Read the model definition and answer for the solid it produces. Units are mm, in the model's axes. A direction names the side the tool comes from. Coordinates: 2 decimals unless noted, no trailing zeros. Loops run counter-clockwise (first coordinate to the right, second up) from the corner with the lowest first, then second, coordinate; pieces in that order, holes last. Notation, with made-up numbers: (-32.5, 21.5) -> (-0.5, 21.5) arc R11 ccw to (-0.5, 30.5) -> close; hole circle Ø10 at (-27, 83). An arc over 180 degrees is marked (long way). Answer as a JSON object with one key per item and string values. Group by question number.
1) Which of the six approach directions +Z, -Z, +X, -X, +Y, -Y give full straight-line access (tool end or side, diameter ignored) to faces 1 (the face through (-72.52, -15, -21)), 2 (the face through (-76, -30, -42))?
2) Determine the mould class of faces 3 (the face through (-25.396, -15, -12)), 4 (the face through (-72.77, -14.79, -11.72)), 5 (the face through (-14.987, -15, -43)), 6 (the face through (-134.987, -15, -43)) for opening direction X: released by +X, released by -X, zero draft, split by the parting line, or undercut.
3) Section A-A, the plane x = -47 is taken. Give the vertices of the cut face in (y, z), plus the area to 3 significant figures.
4) Consider probe 1 along Z at (x, y) = (-119, -21.5); probe 2 along Z at (x, y) = (-49, -6); probe 3 along Z at (x, y) = (-87.5, -7.5). Determine where each line is inside the solid, lowest interval first. Write a range as [from, to].
5) Section B-B, the plane y = -4.5 is taken. Count the separate pieces of the cut face and the enclosed holes in it, plus the area to 3 significant figures.
from build123d import *

# Parameters (mm, degrees)
F0_W     = 120
F0_H     = 85
F0_W_2   = 6.2300768045
F0_H_2   = 1.9291306924
F1_DEPTH = 30


with BuildPart() as f1:
    # F0 (on Front) → F1 (new body)
    with BuildSketch(Plane.XZ):
        with Locations((-74.9865994975, -42.5)):
            Rectangle(F0_W, F0_H)
        with BuildLine():
            Line((-121.3085489491, -24.3586543947), (-121.3085489491, -5.8024477979))
            Line((-121.3085489491, -5.8024477979), (-116.0653747936, -5.8024477979))
            add(Edge.make_bspline(
                [(-116.0653747936, -5.8024477979), (-112.3736278476, -5.8024477979), (-110.7226981077, -6.9071289523)],
                knots=[0, 0, 0, 1, 1, 1], degree=2))
            add(Edge.make_bspline(
                [(-110.7226981077, -6.9071289523), (-109.0717683678, -8.0118101066), (-109.0717683678, -10.3958095096)],
                knots=[0, 0, 0, 1, 1, 1], degree=2))
            add(Edge.make_bspline(
                [(-109.0717683678, -10.3958095096), (-109.0717683678, -12.0487699134), (-109.9916591084, -13.1209604456)],
                knots=[0, 0, 0, 1, 1, 1], degree=2))
            add(Edge.make_bspline(
                [(-109.9916591084, -13.1209604456), (-110.9115498491, -14.1931509778), (-112.6782274306, -14.5099345441)],
                knots=[0, 0, 0, 1, 1, 1], degree=2))
            Line((-112.6782274306, -14.5099345441), (-112.6782274306, -14.6358357051))
            add(Edge.make_bspline(
                [(-112.6782274306, -14.6358357051), (-108.4503852184, -15.3587520488), (-108.4503852184, -19.0789282893)],
                knots=[0, 0, 0, 1, 1, 1], degree=2))
            add(Edge.make_bspline(
                [(-108.4503852184, -19.0789282893), (-108.4503852184, -21.5644608866), (-110.1317749166, -22.9615576407)],
                knots=[0, 0, 0, 1, 1, 1], degree=2))
            add(Edge.make_bspline(
                [(-110.1317749166, -22.9615576407), (-111.8131646148, -24.3586543947), (-114.8347924783, -24.3586543947)],
                knots=[0, 0, 0, 1, 1, 1], degree=2))
            Line((-114.8347924783, -24.3586543947), (-121.3085489491, -24.3586543947))
        make_face(mode=Mode.SUBTRACT)
        with BuildLine():
            add(Edge.make_bspline(
                [(-94.4976936528, -12.1360884606), (-92.7777213407, -14.0794338002), (-92.7777213407, -17.3894159355)],
                knots=[0, 0, 0, 1, 1, 1], degree=2))
            add(Edge.make_bspline(
                [(-92.7777213407, -17.3894159355), (-92.7777213407, -20.7928086097), (-94.4895709972, -22.7036633271)],
                knots=[0, 0, 0, 1, 1, 1], degree=2))
            add(Edge.make_bspline(
                [(-94.4895709972, -22.7036633271), (-96.2014206537, -24.6145180445), (-99.2230485172, -24.6145180445)],
                knots=[0, 0, 0, 1, 1, 1], degree=2))
            add(Edge.make_bspline(
                [(-99.2230485172, -24.6145180445), (-101.0912592929, -24.6145180445), (-102.5370919803, -23.7372712454)],
                knots=[0, 0, 0, 1, 1, 1], degree=2))
            add(Edge.make_bspline(
                [(-102.5370919803, -23.7372712454), (-103.9829246676, -22.8600244463), (-104.7708222557, -21.2233093536)],
                knots=[0, 0, 0, 1, 1, 1], degree=2))
            add(Edge.make_bspline(
                [(-104.7708222557, -21.2233093536), (-105.5587198437, -19.5865942609), (-105.5587198437, -17.3894159355)],
                knots=[0, 0, 0, 1, 1, 1], degree=2))
            add(Edge.make_bspline(
                [(-105.5587198437, -17.3894159355), (-105.5587198437, -13.9900845891), (-103.8570235067, -12.0914138551)],
                knots=[0, 0, 0, 1, 1, 1], degree=2))
            add(Edge.make_bspline(
                [(-103.8570235067, -12.0914138551), (-102.1553271696, -10.192743121), (-99.1336993061, -10.192743121)],
                knots=[0, 0, 0, 1, 1, 1], degree=2))
            add(Edge.make_bspline(
                [(-99.1336993061, -10.192743121), (-96.2176659648, -10.192743121), (-94.4976936528, -12.1360884606)],
                knots=[0, 0, 0, 1, 1, 1], degree=2))
        make_face(mode=Mode.SUBTRACT)
        with BuildLine():
            Line((-78.9651455832, -24.3586543947), (-80.528756776, -24.3586543947))
            Line((-80.528756776, -24.3586543947), (-80.9470735367, -22.3767264413))
            Line((-80.9470735367, -22.3767264413), (-81.048606731, -22.3767264413))
            add(Edge.make_bspline(
                [(-81.048606731, -22.3767264413), (-82.088306641, -23.6844739844), (-83.1219145593, -24.1494960144)],
                knots=[0, 0, 0, 1, 1, 1], degree=2))
            add(Edge.make_bspline(
                [(-83.1219145593, -24.1494960144), (-84.1555224777, -24.6145180445), (-85.7069496871, -24.6145180445)],
                knots=[0, 0, 0, 1, 1, 1], degree=2))
            add(Edge.make_bspline(
                [(-85.7069496871, -24.6145180445), (-87.7741655238, -24.6145180445), (-88.9478892503, -23.5463888401)],
                knots=[0, 0, 0, 1, 1, 1], degree=2))
            add(Edge.make_bspline(
                [(-88.9478892503, -23.5463888401), (-90.1216129769, -22.4782596356), (-90.1216129769, -20.5125769933)],
                knots=[0, 0, 0, 1, 1, 1], degree=2))
            add(Edge.make_bspline(
                [(-90.1216129769, -20.5125769933), (-90.1216129769, -16.3009800922), (-83.3838702007, -16.0979137036)],
                knots=[0, 0, 0, 1, 1, 1], degree=2))
            Line((-83.3838702007, -16.0979137036), (-81.0242387644, -16.0207484759))
            Line((-81.0242387644, -16.0207484759), (-81.0242387644, -15.1556856601))
            add(Edge.make_bspline(
                [(-81.0242387644, -15.1556856601), (-81.0242387644, -13.5189705674), (-81.7268484692, -12.7391956349)],
                knots=[0, 0, 0, 1, 1, 1], degree=2))
            add(Edge.make_bspline(
                [(-81.7268484692, -12.7391956349), (-82.429458174, -11.9594207024), (-83.9808853834, -11.9594207024)],
                knots=[0, 0, 0, 1, 1, 1], degree=2))
            add(Edge.make_bspline(
                [(-83.9808853834, -11.9594207024), (-85.7191336705, -11.9594207024), (-87.9122506681, -13.0234885791)],
                knots=[0, 0, 0, 1, 1, 1], degree=2))
            Line((-87.9122506681, -13.0234885791), (-88.5620631119, -11.411141453))
            add(Edge.make_bspline(
                [(-88.5620631119, -11.411141453), (-87.5345471852, -10.854739548), (-86.3100568615, -10.5379559817)],
                knots=[0, 0, 0, 1, 1, 1], degree=2))
            add(Edge.make_bspline(
                [(-86.3100568615, -10.5379559817), (-85.0855665378, -10.2211724154), (-83.8509228947, -10.2211724154)],
                knots=[0, 0, 0, 1, 1, 1], degree=2))
            add(Edge.make_bspline(
                [(-83.8509228947, -10.2211724154), (-81.3653902973, -10.2211724154), (-80.1652679403, -11.3238229059)],
                knots=[0, 0, 0, 1, 1, 1], degree=2))
            add(Edge.make_bspline(
                [(-80.1652679403, -11.3238229059), (-78.9651455832, -12.4264733964), (-78.9651455832, -14.8632700604)],
                knots=[0, 0, 0, 1, 1, 1], degree=2))
            Line((-78.9651455832, -14.8632700604), (-78.9651455832, -24.3586543947))
        make_face(mode=Mode.SUBTRACT)
        with BuildLine():
            add(Edge.make_bspline(
                [(-70.6800369254, -10.9298741119), (-69.5875397543, -10.192743121), (-68.2797922113, -10.192743121)],
                knots=[0, 0, 0, 1, 1, 1], degree=2))
            add(Edge.make_bspline(
                [(-68.2797922113, -10.192743121), (-67.3538094789, -10.192743121), (-66.618709152, -10.3470735764)],
                knots=[0, 0, 0, 1, 1, 1], degree=2))
            Line((-66.618709152, -10.3470735764), (-66.9111247516, -12.3005722354))
            add(Edge.make_bspline(
                [(-66.9111247516, -12.3005722354), (-67.7721262396, -12.10968983), (-68.4341226667, -12.10968983)],
                knots=[0, 0, 0, 1, 1, 1], degree=2))
            add(Edge.make_bspline(
                [(-68.4341226667, -12.10968983), (-70.1236350204, -12.10968983), (-71.3217267136, -13.4803879536)],
                knots=[0, 0, 0, 1, 1, 1], degree=2))
            add(Edge.make_bspline(
                [(-71.3217267136, -13.4803879536), (-72.5198184068, -14.8510860771), (-72.5198184068, -16.8939339472)],
                knots=[0, 0, 0, 1, 1, 1], degree=2))
            Line((-72.5198184068, -16.8939339472), (-72.5198184068, -24.3586543947))
            Line((-72.5198184068, -24.3586543947), (-74.6276475212, -24.3586543947))
            Line((-74.6276475212, -24.3586543947), (-74.6276475212, -10.4486067707))
            Line((-74.6276475212, -10.4486067707), (-72.8893992342, -10.4486067707))
            Line((-72.8893992342, -10.4486067707), (-72.6457195677, -13.0234885791))
            Line((-72.6457195677, -13.0234885791), (-72.5441863734, -13.0234885791))
            add(Edge.make_bspline(
                [(-72.5441863734, -13.0234885791), (-71.7725340965, -11.6670051027), (-70.6800369254, -10.9298741119)],
                knots=[0, 0, 0, 1, 1, 1], degree=2))
        make_face(mode=Mode.SUBTRACT)
        with Locations((-46.1374331905, -17.3914465994)):
            Rectangle(F0_W_2, F0_H_2, mode=Mode.SUBTRACT)
        with BuildLine():
            Line((-54.2682113929, -24.3586543947), (-54.5484430093, -22.4945049467))
            Line((-54.5484430093, -22.4945049467), (-54.6621601869, -22.4945049467))
            add(Edge.make_bspline(
                [(-54.6621601869, -22.4945049467), (-56.1201768576, -24.6145180445), (-59.0280875434, -24.6145180445)],
                knots=[0, 0, 0, 1, 1, 1], degree=2))
            add(Edge.make_bspline(
                [(-59.0280875434, -24.6145180445), (-61.7572998071, -24.6145180445), (-63.2742057305, -22.7483379326)],
                knots=[0, 0, 0, 1, 1, 1], degree=2))
            add(Edge.make_bspline(
                [(-63.2742057305, -22.7483379326), (-64.7911116539, -20.8821578207), (-64.7911116539, -17.4422131966)],
                knots=[0, 0, 0, 1, 1, 1], degree=2))
            add(Edge.make_bspline(
                [(-64.7911116539, -17.4422131966), (-64.7911116539, -14.0022685725), (-63.2681137389, -12.0975058467)],
                knots=[0, 0, 0, 1, 1, 1], degree=2))
            add(Edge.make_bspline(
                [(-63.2681137389, -12.0975058467), (-61.7451158238, -10.192743121), (-59.0280875434, -10.192743121)],
                knots=[0, 0, 0, 1, 1, 1], degree=2))
            add(Edge.make_bspline(
                [(-59.0280875434, -10.192743121), (-56.1973420853, -10.192743121), (-54.6865281536, -12.2518363021)],
                knots=[0, 0, 0, 1, 1, 1], degree=2))
            Line((-54.6865281536, -12.2518363021), (-54.5200137149, -12.2518363021))
            Line((-54.5200137149, -12.2518363021), (-54.6093629259, -11.2486883421))
            Line((-54.6093629259, -11.2486883421), (-54.6621601869, -10.2699083487))
            Line((-54.6621601869, -10.2699083487), (-54.6621601869, -4.6084174325))
            Line((-54.6621601869, -4.6084174325), (-52.5543310725, -4.6084174325))
            Line((-52.5543310725, -4.6084174325), (-52.5543310725, -24.3586543947))
            Line((-52.5543310725, -24.3586543947), (-54.2682113929, -24.3586543947))
        make_face(mode=Mode.SUBTRACT)
        with BuildLine():
            Line((-27.5527972992, -5.8024477979), (-25.3962322515, -5.8024477979))
            Line((-25.3962322515, -5.8024477979), (-25.3962322515, -17.8077326962))
            add(Edge.make_bspline(
                [(-25.3962322515, -17.8077326962), (-25.3962322515, -20.983691015), (-27.3131789606, -22.7991045297)],
                knots=[0, 0, 0, 1, 1, 1], degree=2))
            add(Edge.make_bspline(
                [(-27.3131789606, -22.7991045297), (-29.2301256696, -24.6145180445), (-32.5807210827, -24.6145180445)],
                knots=[0, 0, 0, 1, 1, 1], degree=2))
            add(Edge.make_bspline(
                [(-32.5807210827, -24.6145180445), (-35.9313164958, -24.6145180445), (-37.7650059855, -22.7848898825)],
                knots=[0, 0, 0, 1, 1, 1], degree=2))
            add(Edge.make_bspline(
                [(-37.7650059855, -22.7848898825), (-39.5986954752, -20.9552617206), (-39.5986954752, -17.7589967629)],
                knots=[0, 0, 0, 1, 1, 1], degree=2))
            Line((-39.5986954752, -17.7589967629), (-39.5986954752, -5.8024477979))
            Line((-39.5986954752, -5.8024477979), (-37.4380690998, -5.8024477979))
            Line((-37.4380690998, -5.8024477979), (-37.4380690998, -17.9092658905))
            add(Edge.make_bspline(
                [(-37.4380690998, -17.9092658905), (-37.4380690998, -20.2323453769), (-36.1689041706, -21.4771423395)],
                knots=[0, 0, 0, 1, 1, 1], degree=2))
            add(Edge.make_bspline(
                [(-36.1689041706, -21.4771423395), (-34.8997392414, -22.721939302), (-32.4385746106, -22.721939302)],
                knots=[0, 0, 0, 1, 1, 1], degree=2))
            add(Edge.make_bspline(
                [(-32.4385746106, -22.721939302), (-30.0911271576, -22.721939302), (-28.8219622284, -21.4710503478)],
                knots=[0, 0, 0, 1, 1, 1], degree=2))
            add(Edge.make_bspline(
                [(-28.8219622284, -21.4710503478), (-27.5527972992, -20.2201613936), (-27.5527972992, -17.8848979239)],
                knots=[0, 0, 0, 1, 1, 1], degree=2))
            Line((-27.5527972992, -17.8848979239), (-27.5527972992, -5.8024477979))
        make_face(mode=Mode.SUBTRACT)
    extrude(amount=F1_DEPTH)


solid = f1.part
Determined:
{
 "1": {"face 1": "+Y, -Y", "face 2": "+Z, -Z, +X, -X, -Y"},
 "2": {"face 3": "undercut", "face 4": "undercut", "face 5": "released by +X", "face 6": "released by -X"},
 "3": {"outline": "(-30, -85) -> (0, -85) -> (0, -18.36) -> (-30, -18.36) -> close; (-30, -16.43) -> (0, -16.43) -> (0, 0) -> (-30, 0) -> close", "area": "2,490 mm²"},
 "4": {"probe 1": "[-85, -24.36], [-5.8, 0]", "probe 2": "[-85, -18.36], [-16.43, 0]", "probe 3": "[-85, -24.36], [-16.82, -12.83], [-10.92, 0]"},
 "5": {"separate pieces": "1", "enclosed holes": "7", "area": "9,420 mm²"}
}
